Verification items for the finished model (mm, model axes). A direction names the side the tool comes from. Round coordinates to 2 decimals unless told otherwise and drop trailing zeros. Write each loop counter-clockwise with the first axis right and the second up, starting at its lowest first coordinate (ties: lowest second). Pieces come first, ordered by that corner, then holes. Notation, with made-up numbers: M 20.5,-28.75 L 77.5,-28.75 A16 ccw 77.5,-9.75 Z; hole C 22.25,51 d8. An arc over 180 degrees is marked long. Answer in a Markdown table with one row per item. Add a question column.
1. Sectioned sample at C-C on y = 5. Record the cut outline in (x, z), plus the area to 3 significant figures.
2. Sectioned sample at B-B on z = -0.95. Record the cut outline in (x, y), plus the area to 3 significant figures.
3. Sectioned sample at A-A on x = -0.7. Record the cut outline in (y, z), plus the area to 3 significant figures.
4. Draft check along Y on faces 1 (the flat face through (0, 0, 0)), 2 (the cylindrical face through (-1.01, 24.75, -0.65)), 3 (the cylindrical face through (-0.45, 25.49, -1.43)). Enter one of: pulls with the +Y half, pulls with the -Y half, needs draft (parallel to the pull), parting line crosses it, or undercut.
5. Set-up check for faces 4 (the cylindrical face through (-1.01, 1.25, -0.65)), 5 (the flat face through (0, 26, 0)): record each of +Z, -Z, +X, -X, +Y, -Y from which the full face is reachable in a straight line by a thin tool's end or side.
6. Material ranges on probe 1 along Y at (x, z) = (-0.65, 1.2); probe 2 along X at (y, z) = (1.75, -1.35); probe 3 along Z at (x, y) = (-0.5, 11.5), recorded low to high.
```python
from build123d import *

# Parameters (mm, degrees)
SKETCH1_R           = 1.5
BOSS_EXTRUDE1_DEPTH = 26
SKETCH2_W           = 2.6975544
SKETCH2_H           = 0.5


with BuildPart() as part:
    # Sketch1 → Boss-Extrude1 (new body)
    with BuildSketch(Plane(origin=(0, 0, 0), x_dir=(1, 0, 0), z_dir=(0, 1, 0))):
        with Locations(Location((0, 0, 0), (0, 0, 90))):
            Circle(SKETCH1_R)
    extrude(amount=BOSS_EXTRUDE1_DEPTH)

    # Sketch2 → Cut-Revolve1 (revolve, cut)
    with BuildSketch(Plane(origin=(0, 0, 0), x_dir=(0, 0, -1), z_dir=(1, 0, 0)), mode=Mode.PRIVATE) as cut_revolve1_sk:
        with Locations((-2.5487772, 1.25)):
            Rectangle(SKETCH2_W, SKETCH2_H)
    cut_revolve1 = revolve(cut_revolve1_sk.sketch.rotate(Axis((0, 0, 0), (0, 1, 0)), 180), axis=Axis((0, 0, 0), (0, 1, 0)), mode=Mode.SUBTRACT)

    # Mirror1: Cut-Revolve1 across plane
    add(cut_revolve1.mirror(Plane.ZX.offset(13)), mode=Mode.SUBTRACT)


solid = part.part
```
Geometry check:
| question | item | result |
|---|---|---|
| 1 | outline | C 0,0 d3 |
| 1 | area | 7.07 mm2 |
| 2 | outline | M -1.16,0 L 1.16,0 L 1.16,1 L 0.73,1 L 0.73,1.5 L 1.16,1.5 L 1.16,24.5 L 0.73,24.5 L 0.73,25 L 1.16,25 L 1.16,26 L -1.16,26 L -1.16,25 L -0.73,25 L -0.73,24.5 L -1.16,24.5 L -1.16,1.5 L -0.73,1.5 L -0.73,1 L -1.16,1 Z |
| 2 | area | 59.5 mm2 |
| 3 | outline | M 0,-1.33 L 1,-1.33 L 1,-0.97 L 1.5,-0.97 L 1.5,-1.33 L 24.5,-1.33 L 24.5,-0.97 L 25,-0.97 L 25,-1.33 L 26,-1.33 L 26,1.33 L 25,1.33 L 25,0.97 L 24.5,0.97 L 24.5,1.33 L 1.5,1.33 L 1.5,0.97 L 1,0.97 L 1,1.33 L 0,1.33 Z |
| 3 | area | 68.3 mm2 |
| 4 | face 1 | pulls with the -Y half |
| 4 | face 2 | undercut |
| 4 | face 3 | needs draft |
| 5 | face 4 | none |
| 5 | face 5 | +Z, -Z, +X, -X, +Y |
| 6 | probe 1 | y = 0 to 1, 1.5 to 24.5, 25 to 26 |
| 6 | probe 2 | x = -0.65 to 0.65 |
| 6 | probe 3 | z = -1.41 to 1.41 |
